from build123d import *

# Parameters (mm, degrees)
F1_DEPTH = 19.304
F2_R     = 20
F3_DEPTH = 15


with BuildPart() as f1:
    # F0 (on Top) → F1 (new body)
    with BuildSketch(Plane.XY):
        with BuildLine():
            ThreePointArc((52.077811, 39.231941), (7.140875, 64.836505), (-41.060608, 46.087135))
            Line((-41.060608, 46.087135), (-37.354928, -29.32171))
            Line((-37.354928, -29.32171), (27.672678, -29.32171))
            Line((27.672678, -29.32171), (52.077811, 39.231941))
        make_face()
    extrude(amount=F1_DEPTH)

    # F2 (on face) → F3 (cut)
    with BuildSketch(Plane.XY.offset(19.304)):
        with Locations((0.727693, 10.67829)):
            Circle(F2_R)
    extrude(amount=-F3_DEPTH, mode=Mode.SUBTRACT)


solid = f1.part
Read the model definition and answer for the solid it produces. Units are mm, in the model's axes. A direction names the side the tool comes from. Round coordinates to 2 decimals unless told otherwise and drop trailing zeros. Order: outer loops, then holes, each group sorted by start corner. A loop starts at its lowest first (then second) coordinate and runs counter-clockwise, first axis right, second up.
1) The part is cut by section A-A on y = 0.5. Write down the section's boundary in (x, z).
2) The part is cut by section C-C on z = 2.25. Write down the section's boundary in (x, y), plus the area to 3 significant figures.
3) Flat-ended cylindrical pins translate along their axes: pin 1 (20 mm diameter, centred on x = 3, y = 10.5, fed in from +Z); pin 2 (3 mm diameter, centred on y = 34, z = 17.5, fed in from +X); pin 3 (5 mm diameter, centred on y = -13, z = 4, fed in from -X). Find the tip coordinate at first contact, or state that the pin passes through.
4) For faces 1 (the face through (5, 18, 0)), 2 (the face through (19.8, 16.7, 11.9)), determine the directions among +Z, -Z, +X, -X, +Y, -Y from which every point of the face is accessible in a straight line to the end or side of a thin tool.
5) The part is cut by section B-B on x = -4. Write down the section's boundary in (y, z), plus the area to 3 significant figures.
6) The part is cut by section D-D on z = 15. Write down the section's boundary in (x, y).
7) The mould has two halves that part along X. Classify faces 3 (the face through (7.887, 64.777, 9.517)), 4 (the face through (15, 29, 19.304)), 5 (the face through (0, 11, 4.304)): released by +X, released by -X, zero draft, split by the parting line, or undercut.
8) Straight lines are drawn through the part: L1, parallel to X at y = 8.5, z = 8; L2, parallel to Y at x = 3.5, z = 13.25; L3, parallel to Y at x = 19, z = 7.75. For each, find the intervals that lie inside material, in ascending order.
Resolved:
1. outline: (-38.82, 0) - (38.29, 0) - (38.29, 19.3) - (17.94, 19.3) - (17.94, 4.3) - (-16.49, 4.3) - (-16.49, 19.3) - (-38.82, 19.3) - close
2. outline: (-41.06, 46.09) - (-37.35, -29.32) - (27.67, -29.32) - (52.08, 39.23) arc R60.15 ccw to start
2. area: 7,170 mm2
3. pin 1: stops at z = 4.3
3. pin 2: stops at x = 50.75
3. pin 3: stops at x = -38.28
4. face 1: -Z, +X, -X, +Y, -Y
4. face 2: +Z
5. outline: (-29.32, 0) - (64.62, 0) - (64.62, 19.3) - (30.11, 19.3) - (30.11, 4.3) - (-8.75, 4.3) - (-8.75, 19.3) - (-29.32, 19.3) - close
5. area: 1,230 mm2
6. outline: (-41.06, 46.09) - (-37.35, -29.32) - (27.67, -29.32) - (52.08, 39.23) arc R60.15 ccw to start; hole circle Ø40 at (0.73, 10.68)
7. face 3: split by the parting line
7. face 4: zero draft
7. face 5: undercut
8. L1: x = -39.21 to -19.15, 20.61 to 41.14
8. L2: y = -29.32 to -9.13, 30.49 to 64.99
8. L3: y = -29.32 to 2.55, 18.81 to 62.76
